Can you work these out from the model? Positions are in its coordinate system, mm. A direction names the side the tool comes from. Give positions to 0.01 mm unless a question says otherwise; leave off trailing zeros. Loops run counter-clockwise (first coordinate to the right, second up) from the corner with the lowest first, then second, coordinate; pieces in that order, holes last. Notation, with made-up numbers: (50.25, -1) - (64.25, -1) arc R10 cw to (64.25, 14) - close; hole circle Ø5 at (-6.75, 60). An arc over 180 degrees is marked (long way). Answer in a Markdown table with one row per item.
from build123d import *

# Parameters (mm, degrees)
SKETCH1_R           = 1.5
BOSS_EXTRUDE3_DEPTH = 5
FILLET1_R           = 1
CUT_EXTRUDE2_DEPTH  = 5


with BuildPart() as part:
    # Sketch1 → Boss-Extrude3 (new body)
    with BuildSketch(Plane.XY):
        with BuildLine():
            Line((20.05, 5), (0, 5))
            ThreePointArc((0, 5), (-5, 0), (0, -5))
            Line((0, -5), (22, -5))
            Line((22, -5), (26.72989842, 1.621129525))
            Line((26.72989842, 1.621129525), (39.900164389, 7.036080522))
            Line((39.900164389, 7.036080522), (46.188488025, 4.540007042))
            Line((46.188488025, 4.540007042), (47.352932204, 4.337597171))
            Line((47.352932204, 4.337597171), (48.038244482, 5.300533868))
            Line((48.038244482, 5.300533868), (49.20268866, 5.098123997))
            Line((49.20268866, 5.098123997), (49.888000938, 6.061060693))
            Line((49.888000938, 6.061060693), (51.052445116, 5.858650822))
            Line((51.052445116, 5.858650822), (51.737757394, 6.821587519))
            Line((51.737757394, 6.821587519), (52.902201573, 6.619177648))
            Line((52.902201573, 6.619177648), (53.587513851, 7.582114344))
            Line((53.587513851, 7.582114344), (54.751958029, 7.379704473))
            Line((54.751958029, 7.379704473), (55.437270307, 8.34264117))
            Line((55.437270307, 8.34264117), (53.72608495, 12.504593197))
            Line((53.72608495, 12.504593197), (46.409029503, 15.837507263))
            Line((46.409029503, 15.837507263), (20.05, 5))
        make_face()
        Circle(SKETCH1_R, mode=Mode.SUBTRACT)
        with Locations((22.020705275, 0.206842568)):
            Circle(SKETCH1_R, mode=Mode.SUBTRACT)
    extrude(amount=BOSS_EXTRUDE3_DEPTH)

    # Fillet1
    fillet1_edges = [part.edges().sort_by_distance(p)[0] for p in [
        (22, -5, 2.5),
        (20.05, 5, 2.5),
        (46.409029503, 15.837507263, 2.5),
        (53.72608495, 12.504593197, 2.5),
        (55.437270307, 8.34264117, 2.5),
        (46.188488025, 4.540007042, 2.5),
        (39.900164389, 7.036080522, 2.5),
        (26.72989842, 1.621129525, 2.5),
    ]]
    fillet(fillet1_edges, radius=FILLET1_R)

    # Sketch4 → Cut-Extrude2 (cut)
    with BuildSketch(Plane(origin=(0, 0, 0), x_dir=(-1, 0, 0), z_dir=(0, 0, -1))):
        with BuildLine():
            Line((-16.936286021, -5), (9.167349916, -5))
            Line((9.167349916, -5), (9.167349916, 5))
            Line((9.167349916, 5), (-16.936286021, 5))
            ThreePointArc((-16.936286021, 5), (-11.936286021, 0), (-16.936286021, -5))
        make_face()
    extrude(amount=-CUT_EXTRUDE2_DEPTH, mode=Mode.SUBTRACT)


solid = part.part
Q1. If we mould it in two halves opening along X, with no side actions, what happens to faces 3 (the face through (48.61, 5.2, 2.46)), 4 (the face through (50.131, 14.142, 2.465)), 5 (the face through (33, 6, 0)), 6 (the face through (33.17, 4.27, 2.46))? For each: released by +X, released by -X, zero draft, split by the parting line, or undercut.
Checked values:
| item | result |
|---|---|
| face 3 | undercut |
| face 4 | released by +X |
| face 5 | zero draft |
| face 6 | undercut |
Q2. Imagine slicing it at B-B, the plane x = 48.5. Write out the boundary of the cut face in (y, z).
Checked values:
| item | result |
|---|---|
| outline | (5.22, 0) - (14.89, 0) - (14.89, 5) - (5.22, 5) - close |
Q3. Imagine slicing it at C-C, the plane x = 16. Write out the boundary of the cut face in (y, z).
Checked values:
| item | result |
|---|---|
| outline | (-4.91, 0) - (4.91, 0) - (4.91, 5) - (-4.91, 5) - close |
Q4. Imagine slicing it at A-A, the plane z = 1.9. Write out the boundary of the cut face in (x, y), and give its area (3 significant figures).
Checked values:
| item | result |
|---|---|
| outline | (16.94, -5) - (21.49, -5) arc R1 ccw to (22.3, -4.58) - (26.56, 1.39) arc R1 cw to (27, 1.73) - (39.53, 6.88) arc R1 cw to (40.28, 6.89) - (46.09, 4.58) arc R1 ccw to (46.29, 4.52) - (47.35, 4.34) - (48.04, 5.3) - (49.2, 5.1) - (49.89, 6.06) - (51.05, 5.86) - (51.74, 6.82) - (52.9, 6.62) - (53.59, 7.58) - (54.75, 7.38) - (55.12, 7.89) arc R1 ccw to (55.23, 8.85) - (53.88, 12.14) arc R1 ccw to (53.37, 12.67) - (46.8, 15.66) arc R1 ccw to (46.01, 15.67) - (20.23, 5.08) arc R1 cw to (19.85, 5) - (16.94, 5) arc R5 ccw to start; hole circle Ø3 at (22.02, 0.21) |
| area | 327 mm² |
Q5. On a 3-axis mill with a long thin cutter (end or side, diameter ignored), from which of +Z, -Z, +X, -X, +Y, -Y can I reach the whole of each face in a straight line? I mean faces 1 (the face through (46.81, 4.43, 2.46)), 2 (the face through (24.4, -1.64, 2.46)). Say none if no direction works.
Checked values:
| item | result |
|---|---|
| face 1 | +Z, -Z, -Y |
| face 2 | +Z, -Z, +X, -Y |
Q6. For pin 1 (2.5 mm diameter, centred on x = 19, z = 2.5, fed in from +Y); pin 2 (1.5 mm diameter, centred on x = 42.5, z = 1, fed in from -Y), each with a flat end and sliding along its axis, tell me the tip position at first contact or that it passes through.
Checked values:
| item | result |
|---|---|
| pin 1 | stops at y = 5.08 |
| pin 2 | stops at y = 5.71 |
Q7. If I drill on line 1 (Y direction, x = 19.5, z = 1.95); line 2 (Y direction, x = 23, z = 2.5); line 3 (X direction, y = 3.5, z = 0.6), over which ranges is the centre line in solid material (lowest first)? Write a range as [from, to].
Checked values:
| item | result |
|---|---|
| line 1 | y = [-5, 5] |
| line 2 | y = [-3.6, -0.93], [1.34, 6.21] |
| line 3 | x = [13.37, 31.3] |
